Verification items for the finished model (mm, model axes). A direction names the side the tool comes from. Round coordinates to 2 decimals unless told otherwise and drop trailing zeros. Order: outer loops, then holes, each group sorted by start corner. A loop starts at its lowest first (then second) coordinate and runs counter-clockwise, first axis right, second up. Notation, with made-up numbers: M 47,-6 L 91,-6 A31 cw 91,33 Z; hole C 4,26 d11. An arc over 180 degrees is marked long. Use CSV: the item, a comma, the result in double quotes. Start each with the question number.
Q1. Mould release check, pull along Y, two halves, no side actions. Record for faces 1 (the face through (-10, -69.85, 10)), 2 (the face through (-19.05, 2, 9)), 3 (the face through (0.3, 118.7, 7.7)): +Y half, -Y half, draft (parallel to the pull), parting line (faces both ways), or undercut.
Q2. Scan lines: line 1 (Z direction, x = 4, y = 114); line 2 (Y direction, x = 0.5, z = 9.25); line 3 (Y direction, x = 14.5, z = 12.75). Record each from-to range of solid material in increasing order.
Q3. Set-up check for faces 4 (the face through (6.35, 0, 10)), 5 (the face through (7.77, -98.825, 11.134)), 6 (the face through (0, 2, 0)): record each of +Z, -Z, +X, -X, +Y, -Y from which the full face is reachable in a straight line by a thin tool's end or side.
Q4. Sectioned sample at B-B (y = -57.15). Enter the section's corners in (x, z), and give its area (3 significant figures).
Q5. Sectioned sample at A-A (y = 114.3). Enter the section's corners in (x, z), and give its area (3 significant figures).
Q6. Gauge pin test, flat ends, axial feed: pin 1 Ø8.5 at (y, z) = (-57.15, 9.525) entering from +X; pin 2 Ø8.5 at (y, z) = (114.3, 9.525) entering from +X. Record the tip position at first contact, or that the pin passes through.
Q7. Sectioned sample at C-C (x = 14). State how many separate pieces and enclosed holes the cut face has, and give its area (3 significant figures).
```python
from build123d import *

# Parameters (mm, degrees)
F1_DEPTH = 19.05
F2_R     = 4.7625
F3_DEPTH = 38.101
F4_R     = 2.38125
F5_DEPTH = 57.15
F6_DEPTH = 12.7


with BuildPart() as f1:
    # F0 (on Top) → F1 (new body)
    with BuildSketch(Plane.XY):
        Polygon((19.05, -127), (19.05, 127), (12.7, 127), (-19.05, 63.5), (-19.05, -127), align=None)
        Polygon((-19.05, 63.5), (12.7, 127), (-19.05, 127), align=None)
    extrude(amount=F1_DEPTH)

    # F2 (on face) → F3 (cut, through all)
    with BuildSketch(Plane.YZ.offset(19.05)):
        with Locations((114.3, 9.525)):
            Circle(F2_R)
    extrude(amount=-F3_DEPTH, mode=Mode.SUBTRACT)

    # F4 (on face) → F5 (cut)
    with BuildSketch(Plane.XZ.offset(127)):
        with Locations((-9.525, 9.525)):
            Circle(F4_R)
        with Locations((9.525, 9.525)):
            Circle(F4_R)
    extrude(amount=-F5_DEPTH, mode=Mode.SUBTRACT)

    # F2 (on face) → F6 (cut)
    with BuildSketch(Plane.YZ.offset(19.05)):
        with Locations((-57.15, 9.525)):
            Circle(F2_R)
        with Locations((0, 9.525)):
            Circle(F2_R)
        with Locations((57.15, 9.525)):
            Circle(F2_R)
    extrude(amount=-F6_DEPTH, mode=Mode.SUBTRACT)


solid = f1.part
```
Verdict:
1,face 1,"-Y half"
1,face 2,"draft"
1,face 3,"undercut"
2,line 1,"z = 0 to 4.77, 14.28 to 19.05"
2,line 2,"y = -127 to 109.55, 119.05 to 127"
2,line 3,"y = -127 to -60.65, -53.65 to -3.5, 3.5 to 53.65, 60.65 to 110.8, 117.8 to 127"
3,face 4,"+X"
3,face 5,"-Y"
3,face 6,"-Z, +X, -X, +Y, -Y"
4,outline,"M -19.05,0 L 19.05,0 L 19.05,4.76 L 6.35,4.76 L 6.35,14.29 L 19.05,14.29 L 19.05,19.05 L -19.05,19.05 Z"
4,area,"605 mm²"
5,outline,"M -19.05,0 L 19.05,0 L 19.05,4.76 L -19.05,4.76 Z; M -19.05,14.29 L 19.05,14.29 L 19.05,19.05 L -19.05,19.05 Z"
5,area,"363 mm²"
6,pin 1,"stops at x = 6.35"
6,pin 2,"passes through"
7,separate pieces,"1"
7,enclosed holes,"4"
7,area,"4,550 mm²"
